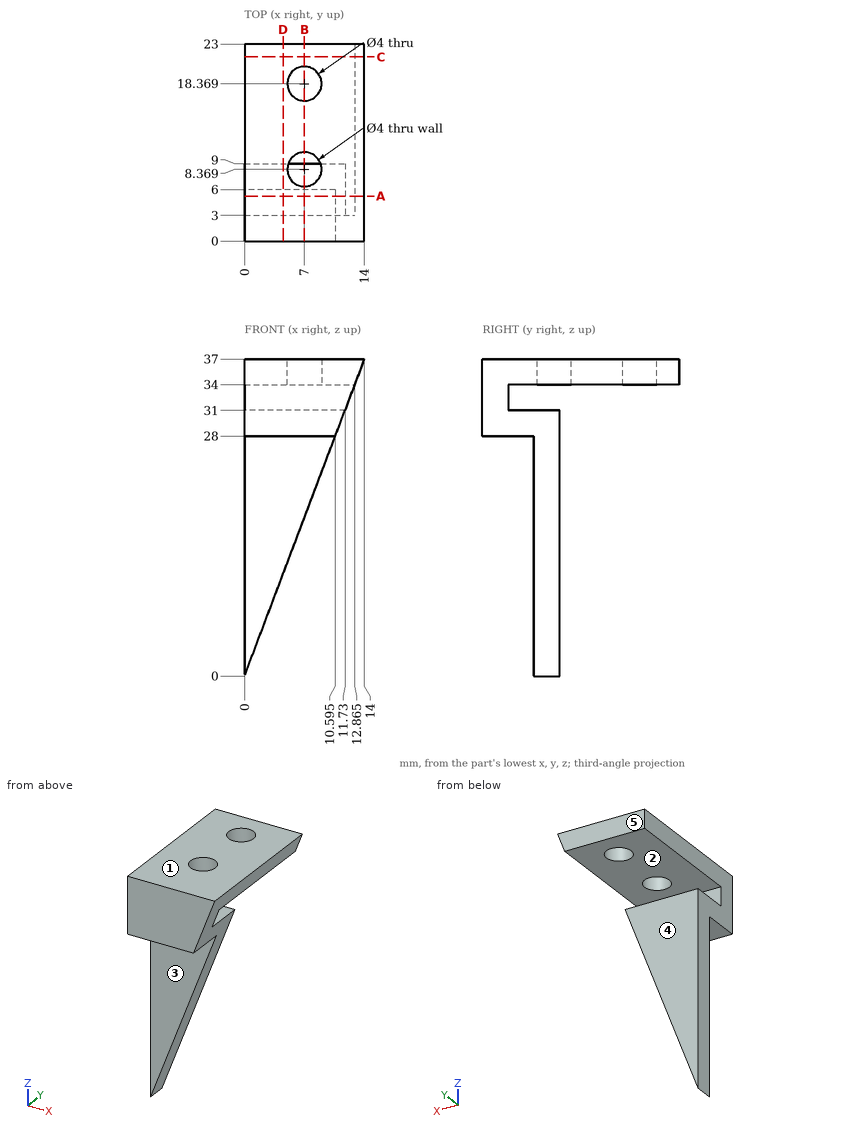
Here's the drawing with two shaded views (mm, measured from the low corner). I have some questions. A direction names the side the tool comes from. Coordinates: 2 decimals unless noted, no trailing zeros. Loops run counter-clockwise (first coordinate to the right, second up) from the corner with the lowest first, then second, coordinate; pieces in that order, holes last. Notation, with made-up numbers: M 22,20.25 L 26,20.25 A26 ccw 26,44.25 Z; hole C 72.25,88.5 d4. An arc over 180 degrees is marked long. Answer as CSV lines item,"result". Start each with the question number.
1. Suppose I cut it at D-D, the plane x = 4.5. List the corners of the cut face in (y, z) for me, plus the area to 3 significant figures.
2. Suppose I cut it at A-A, the plane y = 5.25. List the corners of the cut face in (x, z) for me (1 decimal).
3. For the marked faces 4 and 5, which set-ups out of +Z, -Z, +X, -X, +Y, -Y let a thin tool reach every point of the face, with its end or its side?
4. For pin 1 Ø2 at (x, z) = (10.5, 22) entering from -Y; pin 2 Ø12 at (y, z) = (17.5, 29.5) entering from +X; pin 3 Ø8 at (x, y) = (12.5, 20) entering from -Z; pin 4 Ø10 at (y, z) = (9.5, 20.5) entering from +X, each with a flat end and sliding along its axis, tell me the tip position at first contact or that it passes through.
5. If I drill on probe 1 along Y at (x, z) = (7, 34.9); probe 2 along Z at (x, y) = (9.5, 4); probe 3 along Z at (x, y) = (3.25, 15), over which ranges is the centre line in solid material (lowest first)? Write a range as [from, to].
6. Thinking about a two-plate mould opening in Z: for the marked faces 1, 2 and 3, which applies, +Z half, -Z half, draft (parallel to the pull), parting line (faces both ways), or undercut?
7. Suppose I cut it at B-B, the plane x = 7. List the corners of the cut face in (y, z) for me.
8. Suppose I cut it at C-C, the plane y = 21.5. List the corners of the cut face in (x, z) for me (1 decimal), plus the area to 3 significant figures.
Output:
1,outline,"M 0,28 L 6,28 L 6,11.89 L 9,11.89 L 9,31 L 3,31 L 3,34 L 23,34 L 23,37 L 0,37 Z"
1,area,"153 mm^2"
2,outline,"M 0,28 L 10.6,28 L 11.7,31 L 0,31 Z; M 0,34 L 12.9,34 L 14,37 L 0,37 Z"
3,face 4,"-Z, +X, -X, +Y"
3,face 5,"+Z, -Z, +X, -X, +Y"
4,pin 1,"passes through"
4,pin 2,"stops at x = 13.43"
4,pin 3,"stops at z = 34"
4,pin 4,"stops at x = 9.64"
5,probe 1,"y = [0, 6.37], [10.37, 16.37], [20.37, 23]"
5,probe 2,"z = [28, 31], [34, 37]"
5,probe 3,"z = [34, 37]"
6,face 1,"+Z half"
6,face 2,"undercut"
6,face 3,"draft"
7,outline,"M 0,28 L 6,28 L 6,18.5 L 9,18.5 L 9,31 L 3,31 L 3,34 L 6.37,34 L 6.37,37 L 0,37 Z; M 10.37,34 L 16.37,34 L 16.37,37 L 10.37,37 Z; M 20.37,34 L 23,34 L 23,37 L 20.37,37 Z"
8,outline,"M 0,34 L 12.9,34 L 14,37 L 0,37 Z"
8,area,"40.3 mm^2"
